Autodesk Inventor part; units mm, degrees
ref_plane "YZ Plane" through (0, 0, 0) normal (1, 0, 0) x (0, 1, 0)
ref_plane "XZ Plane" through (0, 0, 0) normal (0, 1, 0) x (-1, 0, 0)
ref_plane "XY Plane" through (0, 0, 0) normal (0, 0, 1) x (1, 0, 0)
sketch "Szkic1" plane through (0, 0, 0) normal (0, 1, 0) x (-1, 0, 0)
  circle A0 centre (0, 0) radius 8
  circle A1 centre (0, 0) radius 12.5
  dimension "d0" = 16
  dimension "d1" = 25
extrude "Wyciągnięcie proste1" add sketch "Szkic1" along normal blind 40
sketch "Szkic2" plane through (0, 0, 0) normal (0, -1, 0) x (1, 0, 0)
  circle A0 centre (0, 0) radius 8
  circle A1 centre (0, 0) radius 8
  circle A2 centre (0, 0) radius 12.5
extrude "Wyciągnięcie proste2" add sketch "Szkic2" against normal blind 20 contours A0
fillet "Zaokrąglenie1" radius 12 1 edges at (12.5, 0, 0)
sketch "Szkic3" plane through (0, 20, 0) normal (0, 1, 0) x (1, 0, 0)
  circle A0 centre (0, 0) radius 8
  line L0 (-4, -4) -> (4, -4)
  line L1 (4, -4) -> (4, 4)
  line L2 (4, 4) -> (-4, 4)
  line L3 (-4, 4) -> (-4, -4)
  line L4 (-4, -4) -> (4, 4) construction
  line L5 (4, -4) -> (-4, 4) construction
  dimension "d7" = 8
  dimension "d8" = 8
extrude "Wyciągnięcie proste3" cut sketch "Szkic3" against normal blind 3.5 contours L3 L2 L1 L0
chamfer "Faza1" distance 0.5 angle 45 4 edges at (4, 20, 0) (0, 20, -4) (0, 20, 4) (-4, 20, 0)
properties part number "koncowka do laski - zaokraglona"
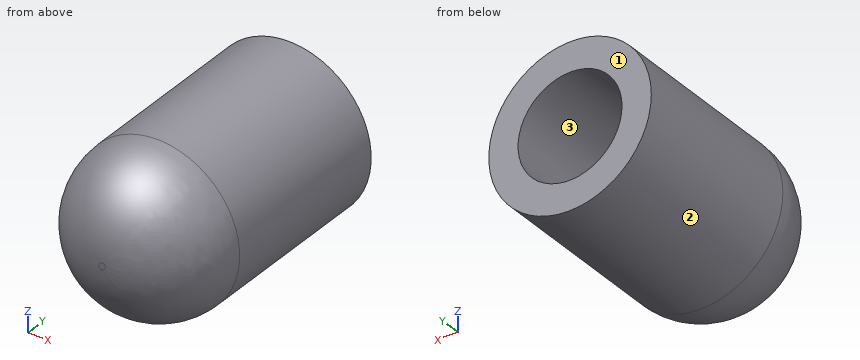
Work out the finished part from the listing and answer in its coordinate system (mm). Face numbers are marked on the shaded views. Give positions to 0.01 mm unless a question says otherwise; leave off trailing zeros. Loops run counter-clockwise (first coordinate to the right, second up) from the corner with the lowest first, then second, coordinate; pieces in that order, holes last. Notation, with made-up numbers: (-30, 22.25) -> (-26, 22.25) arc R20 ccw to (-26, 53.25) -> close; hole circle Ø9 at (-17.5, 31). An arc over 180 degrees is marked (long way). Write item = value, one per line. Start each with the question number.
(1) Find section A-A on y = 27. Give the vertices of the cut face in (x, z).
(2) The mould has two halves that part along Z. Classify the marked faces 1, 2 and 3: +Z half, -Z half, draft (parallel to the pull), parting line (faces both ways), or undercut.
(3) Find the intervals of material crossed by probe 1 along Z at (x, y) = (0, 27.75); probe 2 along X at (y, z) = (23, 4.25); probe 3 along X at (y, z) = (26.5, 5) (3 decimals), in increasing order. Write a range as from..to.
(4) Given pin 1 Ø0.9 at (x, y) = (-1, 18.5) entering from +Z; pin 2 Ø1.5 at (y, z) = (14, -4) entering from -X; pin 3 Ø1.5 at (x, y) = (4, 15) entering from +Z, each flat-ended and moving along its own axis, determine where each tip first touches the part or whether it passes through.
From the geometry:
q1.outline = circle Ø25 at (0, 0); hole circle Ø16 at (0, 0)
q2.face_1 = draft
q2.face_2 = parting line
q2.face_3 = undercut
q3.probe_1 = -12.5..-8, 8..12.5
q3.probe_2 = -11.76..-6.78, 6.78..11.76
q3.probe_3 = -11.456..-6.245, 6.245..11.456
q4.pin_1 = 12.49
q4.pin_2 = -12.07
q4.pin_3 = 12.07
